```python
from build123d import *

# Parameters (mm, degrees)
F0_W           = 95
F0_H           = 40
F1_DEPTH       = 8
F2_D           = 5.5
F2_CBORE_D     = 9.75
F2_CBORE_DEPTH = 4
F3_D           = 13


with BuildPart() as f1:
    # F0 (on Front) → F1 (new body)
    with BuildSketch(Plane.XZ):
        Rectangle(F0_W, F0_H)
    extrude(amount=-F1_DEPTH)

    # F2 (through all)
    with Locations(Plane.XZ):
        with Locations((-17.5, -13), (-37.5, -13)):
            CounterBoreHole(F2_D / 2, F2_CBORE_D / 2, F2_CBORE_DEPTH)

    # F3 (through all)
    with Locations(Plane.XZ):
        with Locations((27.5, 0)):
            Hole(F3_D / 2)


solid = f1.part
```
Build history of the part. All positions in model axes, mm. A direction names the side the tool comes from. Round coordinates to 2 decimals unless told otherwise and drop trailing zeros. Write each loop counter-clockwise with the first axis right and the second up, starting at its lowest first coordinate (ties: lowest second). Pieces come first, ordered by that corner, then holes. Notation, with made-up numbers: (53, 29) -> (105, 29) arc R21 ccw to (105, 53) -> close; hole circle Ø3 at (75.5, 74). An arc over 180 degrees is marked (long way). Put each result on its own line as item: value.
Item 1: Slice it at A-A, the plane z = 0. Give the cut face in (x, y), plus the area to 3 significant figures.
Here are the results:
outline: (-47.5, 0) -> (21, 0) -> (21, 8) -> (-47.5, 8) -> close; (34, 0) -> (47.5, 0) -> (47.5, 8) -> (34, 8) -> close
area: 656 mm^2
Item 2: Slice it at D-D, the plane z = -13. Give the cut face in (x, y) (3 decimals).
Here are the results:
outline: (-47.5, 0) -> (-42.375, 0) -> (-42.375, 4) -> (-40.25, 4) -> (-40.25, 8) -> (-47.5, 8) -> close; (-34.75, 4) -> (-32.625, 4) -> (-32.625, 0) -> (-22.375, 0) -> (-22.375, 4) -> (-20.25, 4) -> (-20.25, 8) -> (-34.75, 8) -> close; (-14.75, 4) -> (-12.625, 4) -> (-12.625, 0) -> (47.5, 0) -> (47.5, 8) -> (-14.75, 8) -> close
Item 3: Wall check: probe 1 along Z at (x, y) = (-37.5, 3.1) (3 decimals); probe 2 along Z at (x, y) = (-37.5, 6.3); probe 3 along X at (y, z) = (6, -14.5). Give the ranges that are in metal, low to high. Write a range as from..to.
Here are the results:
probe 1: z = -20..-17.875, -8.125..20
probe 2: z = -20..-15.75, -10.25..20
probe 3: x = -47.5..-39.8, -35.2..-19.8, -15.2..47.5
Item 4: Two-plate mould, pull along X, no slides. Class faces 1 (the face through (-47.5, 4, 0)), 2 (the face through (-35.25, 1.972, -17.325)), 3 (the face through (-1, 8, 0)), 4 (the face through (-35, 4, -15)): pulls with the +X half, pulls with the -X half, needs draft (parallel to the pull), parting line crosses it, or undercut.
Here are the results:
face 1: pulls with the -X half
face 2: undercut
face 3: needs draft
face 4: undercut
Item 5: Slice it at B-B, the plane x = 27.5. Give the cut face in (y, z), plus the area to 3 significant figures.
Here are the results:
outline: (0, -20) -> (8, -20) -> (8, -6.5) -> (0, -6.5) -> close; (0, 6.5) -> (8, 6.5) -> (8, 20) -> (0, 20) -> close
area: 216 mm^2
Item 6: Tool access for faces 5 (the face through (-15, 4, -15)), 6 (the face through (-34.753, 6.028, -12.879)): list every direction of +Z, -Z, +X, -X, +Y, -Y with a clear straight run to the whole face (end or side of a thin tool).
Here are the results:
face 5: -Y
face 6: +Y, -Y
Item 7: Slice it at C-C, the plane y = 6.5. Give the cut face in (x, z).
Here are the results:
outline: (-47.5, -20) -> (47.5, -20) -> (47.5, 20) -> (-47.5, 20) -> close; hole circle Ø5.5 at (-37.5, -13); hole circle Ø5.5 at (-17.5, -13); hole circle Ø13 at (27.5, 0)
